from build123d import *

# Parameters (mm, degrees)
F1_DEPTH = 2.5
F2_R     = 0.85
F3_DEPTH = 12.5


with BuildPart() as f1:
    # F0 (on Top) → F1 (new body)
    with BuildSketch(Plane.XY):
        with BuildLine():
            Line((13.081475452, -13.081475452), (1.0606601718, -1.0606601718))
            ThreePointArc((1.0606601718, -1.0606601718), (0, -0.6213203436), (-1.0606601718, -1.0606601718))
            Line((-1.0606601718, -1.0606601718), (-13.081475452, -13.081475452))
            ThreePointArc((-13.081475452, -13.081475452), (-13.5208152802, -14.1421356237), (-13.081475452, -15.2027957955))
            Line((-13.081475452, -15.2027957955), (-1.0606601718, -27.2236110757))
            ThreePointArc((-1.0606601718, -27.2236110757), (0, -27.6629509039), (1.0606601718, -27.2236110757))
            Line((1.0606601718, -27.2236110757), (13.081475452, -15.2027957955))
            ThreePointArc((13.081475452, -15.2027957955), (13.5208152802, -14.1421356237), (13.081475452, -13.081475452))
        make_face()
        with BuildLine():
            add(Edge.make_bspline(
                [(-2.6307656823, -7.7655284531), (-3.193916724, -7.5018565781), (-3.7570677656, -7.5018565781)],
                knots=[0, 0, 0, 1, 1, 1], degree=2))
            add(Edge.make_bspline(
                [(-3.7570677656, -7.5018565781), (-4.5741250573, -7.5018565781), (-5.0472153351, -8.0460189045)],
                knots=[0, 0, 0, 1, 1, 1], degree=2))
            add(Edge.make_bspline(
                [(-5.0472153351, -8.0460189045), (-5.5203056128, -8.5901812309), (-5.5203056128, -9.5363617864)],
                knots=[0, 0, 0, 1, 1, 1], degree=2))
            add(Edge.make_bspline(
                [(-5.5203056128, -9.5363617864), (-5.5203056128, -10.5085840087), (-5.0640339115, -11.0397255017)],
                knots=[0, 0, 0, 1, 1, 1], degree=2))
            add(Edge.make_bspline(
                [(-5.0640339115, -11.0397255017), (-4.6077622101, -11.5708669948), (-3.7635781823, -11.5708669948)],
                knots=[0, 0, 0, 1, 1, 1], degree=2))
            add(Edge.make_bspline(
                [(-3.7635781823, -11.5708669948), (-3.2449149878, -11.5708669948), (-2.5797674184, -11.3842350503)],
                knots=[0, 0, 0, 1, 1, 1], degree=2))
            Line((-2.5797674184, -11.3842350503), (-2.5797674184, -11.888792342))
            add(Edge.make_bspline(
                [(-2.5797674184, -11.888792342), (-3.0951754045, -12.0830197725), (-3.8514688073, -12.0830197725)],
                knots=[0, 0, 0, 1, 1, 1], degree=2))
            add(Edge.make_bspline(
                [(-3.8514688073, -12.0830197725), (-4.9463038767, -12.0830197725), (-5.541464467, -11.4178722031)],
                knots=[0, 0, 0, 1, 1, 1], degree=2))
            add(Edge.make_bspline(
                [(-5.541464467, -11.4178722031), (-6.1366250573, -10.7527246337), (-6.1366250573, -9.5287663003)],
                knots=[0, 0, 0, 1, 1, 1], degree=2))
            add(Edge.make_bspline(
                [(-6.1366250573, -9.5287663003), (-6.1366250573, -8.7627072725), (-5.850166724, -8.1865353975)],
                knots=[0, 0, 0, 1, 1, 1], degree=2))
            add(Edge.make_bspline(
                [(-5.850166724, -8.1865353975), (-5.5637083906, -7.6103635225), (-5.0228012726, -7.2984060573)],
                knots=[0, 0, 0, 1, 1, 1], degree=2))
            add(Edge.make_bspline(
                [(-5.0228012726, -7.2984060573), (-4.4818941545, -6.986448592), (-3.7494722795, -6.986448592)],
                knots=[0, 0, 0, 1, 1, 1], degree=2))
            add(Edge.make_bspline(
                [(-3.7494722795, -6.986448592), (-2.9703924184, -6.986448592), (-2.3866250573, -7.2707367864)],
                knots=[0, 0, 0, 1, 1, 1], degree=2))
            Line((-2.3866250573, -7.2707367864), (-2.6307656823, -7.7655284531))
        make_face(mode=Mode.SUBTRACT)
        with BuildLine():
            Line((-8.1334756687, -14.8039748892), (-8.1334756687, -13.4802963582))
            Line((-8.1334756687, -13.4802963582), (-0.6236797201, -13.4802963582))
            Line((-0.6236797201, -13.4802963582), (-0.6236797201, -6.9198086858))
            ThreePointArc((-0.6236797201, -6.9198086858), (-0.9032194318, -6.4583786209), (-0.9135835525, -5.9189782686))
            ThreePointArc((-0.9135835525, -5.9189782686), (0.0168397474, -5.0141534426), (0.9868078824, -5.876451129))
            ThreePointArc((0.9868078824, -5.876451129), (0.9900106564, -6.4384308628), (0.6999988109, -6.9198086858))
            Line((0.6999988109, -6.9198086858), (0.6999988109, -13.4802963582))
            Line((0.6999988109, -13.4802963582), (8.1334756687, -13.4802963582))
            ThreePointArc((8.1334756687, -13.4802963582), (8.5949057336, -13.2007566465), (9.134306086, -13.1903925258))
            ThreePointArc((9.134306086, -13.1903925258), (10.0391309119, -14.1208158258), (9.1768332255, -15.0907839607))
            ThreePointArc((9.1768332255, -15.0907839607), (8.6148534917, -15.0939867347), (8.1334756687, -14.8039748892))
            Line((8.1334756687, -14.8039748892), (0.6999988109, -14.8039748892))
            Line((0.6999988109, -14.8039748892), (0.6999988109, -23.1867600232))
            Line((0.6999988109, -23.1867600232), (-0.6236797201, -23.1867600232))
            Line((-0.6236797201, -23.1867600232), (-0.6236797201, -14.8039748892))
            Line((-0.6236797201, -14.8039748892), (-8.1334756687, -14.8039748892))
        make_face(mode=Mode.SUBTRACT)
        with BuildLine():
            Line((4.5060936962, -9.9324142291), (4.5060936962, -9.417006243))
            Line((4.5060936962, -9.417006243), (6.1912065434, -9.417006243))
            Line((6.1912065434, -9.417006243), (6.1912065434, -11.8280305486))
            add(Edge.make_bspline(
                [(6.1912065434, -11.8280305486), (5.7973263351, -11.9538986041), (5.3904252934, -12.0184602361)],
                knots=[0, 0, 0, 1, 1, 1], degree=2))
            add(Edge.make_bspline(
                [(5.3904252934, -12.0184602361), (4.9835242517, -12.083021868), (4.4474999462, -12.083021868)],
                knots=[0, 0, 0, 1, 1, 1], degree=2))
            add(Edge.make_bspline(
                [(4.4474999462, -12.083021868), (3.3222829323, -12.083021868), (2.6951127934, -11.4129914861)],
                knots=[0, 0, 0, 1, 1, 1], degree=2))
            add(Edge.make_bspline(
                [(2.6951127934, -11.4129914861), (2.0679426545, -10.7429611041), (2.0679426545, -9.5363638819)],
                knots=[0, 0, 0, 1, 1, 1], degree=2))
            add(Edge.make_bspline(
                [(2.0679426545, -9.5363638819), (2.0679426545, -8.762709368), (2.3782725156, -8.1811121458)],
                knots=[0, 0, 0, 1, 1, 1], degree=2))
            add(Edge.make_bspline(
                [(2.3782725156, -8.1811121458), (2.6886023767, -7.5995149236), (3.2718272031, -7.2929828055)],
                knots=[0, 0, 0, 1, 1, 1], degree=2))
            add(Edge.make_bspline(
                [(3.2718272031, -7.2929828055), (3.8550520295, -6.9864506875), (4.637387099, -6.9864506875)],
                knots=[0, 0, 0, 1, 1, 1], degree=2))
            add(Edge.make_bspline(
                [(4.637387099, -6.9864506875), (5.4316579323, -6.9864506875), (6.1163367517, -7.2772492986)],
                knots=[0, 0, 0, 1, 1, 1], degree=2))
            Line((6.1163367517, -7.2772492986), (5.8928124462, -7.786146868))
            add(Edge.make_bspline(
                [(5.8928124462, -7.786146868), (5.2211544601, -7.5018586736), (4.6004947378, -7.5018586736)],
                knots=[0, 0, 0, 1, 1, 1], degree=2))
            add(Edge.make_bspline(
                [(4.6004947378, -7.5018586736), (3.6955468212, -7.5018586736), (3.1866492517, -8.0405956527)],
                knots=[0, 0, 0, 1, 1, 1], degree=2))
            add(Edge.make_bspline(
                [(3.1866492517, -8.0405956527), (2.6777516823, -8.5793326319), (2.6777516823, -9.5363638819)],
                knots=[0, 0, 0, 1, 1, 1], degree=2))
            add(Edge.make_bspline(
                [(2.6777516823, -9.5363638819), (2.6777516823, -10.540053118), (3.1676605365, -11.0587163125)],
                knots=[0, 0, 0, 1, 1, 1], degree=2))
            add(Edge.make_bspline(
                [(3.1676605365, -11.0587163125), (3.6575693906, -11.5773795069), (4.6070051545, -11.5773795069)],
                knots=[0, 0, 0, 1, 1, 1], degree=2))
            add(Edge.make_bspline(
                [(4.6070051545, -11.5773795069), (5.1224131406, -11.5773795069), (5.613949599, -11.458021868)],
                knots=[0, 0, 0, 1, 1, 1], degree=2))
            Line((5.613949599, -11.458021868), (5.613949599, -9.9324142291))
            Line((5.613949599, -9.9324142291), (4.5060936962, -9.9324142291))
        make_face(mode=Mode.SUBTRACT)
    extrude(amount=F1_DEPTH)

    # F2 (on Right) → F3 (cut, symmetric)
    with BuildSketch(Plane.YZ):
        with Locations((-2.4908210296, 1.292226194)):
            Circle(F2_R)
    extrude(amount=F3_DEPTH, both=True, mode=Mode.SUBTRACT)


solid = f1.part
Can you work these out from the model? Positions are in its coordinate system, mm. A direction names the side the tool comes from. Give positions to 0.01 mm unless a question says otherwise; leave off trailing zeros. Loops run counter-clockwise (first coordinate to the right, second up) from the corner with the lowest first, then second, coordinate; pieces in that order, holes last. Notation, with made-up numbers: (28, -34.5) - (61, -34.5) arc R15 cw to (61, -7.5) - close; hole circle Ø2 at (-30, -34). An arc over 180 degrees is marked (long way). Answer as a JSON object with one key per item and string values.
Q1. Which directions (+Z, -Z, +X, -X, +Y, -Y) give clear straight access to the entire face, cutting with the end or side of a thin tool? Please do faces 1 (the flat face through (-4, -14.804, 1)), 2 (the cylindrical face through (-13.52, -14.13, 1.23)).
Geometry says:
{"face 1": "+Z, -Z", "face 2": "+Z, -Z, -X"}
Q2. If I drill on L1, parallel to X at y = -8.5, z = 1.8; L2, parallel to Y at x = -0.75, z = 0.8; L3, parallel to X at y = -8.25, z = 0.6, over which ranges is the centre line in solid material (lowest first)?
Geometry says:
{"L1": "-8.5 to -5.98, -5.33 to -0.62, 0.7 to 2.24, 2.88 to 8.5", "L2": "-27.46 to -14.8, -13.48 to -6.77, -5.43 to -3.18, -1.8 to -0.82", "L3": "-8.25 to -5.88, -5.2 to -0.62, 0.7 to 2.34, 3.02 to 8.25"}
Q3. Imagine slicing it at B-B on x = -7. Write out the boundary of the cut face in (y, z).
Geometry says:
{"outline": "(-21.28, 0) - (-14.8, 0) - (-14.8, 2.5) - (-21.28, 2.5) - close; (-13.48, 0) - (-7, 0) - (-7, 2.5) - (-13.48, 2.5) - close"}
Q4. If we mould it in two halves opening along X, with no side actions, what happens to faces 3 (the flat face through (-1, -16, 0)), 4 (the cylindrical face through (-0.016, -27.663, 1.232)), 5 (the cylindrical face through (1, -6.4, 1.2))? For each: pulls with the +X half, pulls with the -X half, needs draft (parallel to the pull), parting line crosses it, or undercut.
Geometry says:
{"face 3": "needs draft", "face 4": "parting line crosses it", "face 5": "undercut"}
Q5. Imagine slicing it at C-C on z = 0.8. Give the number of separate pieces and of enclosed holes in the cut face, plus the area to 3 significant figures.
Geometry says:
{"separate pieces": "2", "enclosed holes": "3", "area": "331 mm²"}
Q6. Will these pins go through, and if not, where does the flat tip stop? P1, Ø1.5, axis at x = 4.5, z = 1, coming from the -Y side; P2, Ø0.5, axis at x = 5.5, z = 1.5, coming from the -Y side; P3, Ø0.6, axis at x = 5, z = 1, coming from the +Y side.
Geometry says:
{"P1": "y = -24.53", "P2": "y = -23.03", "P3": "y = -4.7"}
Q7. Imagine slicing it at A-A on y = -2.75. Write out the boundary of the cut face in (x, z), plus the area to 3 significant figures.
Geometry says:
{"outline": "(-2.75, 0) - (2.75, 0) - (2.75, 0.48) - (-2.75, 0.48) - close; (-2.75, 2.1) - (2.75, 2.1) - (2.75, 2.5) - (-2.75, 2.5) - close", "area": "4.85 mm²"}
